Design review of the part built by this model. Coordinates are the model's own, in mm. A direction names the side the tool comes from. Give positions to 0.01 mm unless a question says otherwise; leave off trailing zeros. Loops run counter-clockwise (first coordinate to the right, second up) from the corner with the lowest first, then second, coordinate; pieces in that order, holes last. Notation, with made-up numbers: (-15, -11) -> (5, -11) arc R36 ccw to (5, 28) -> close; hole circle Ø2 at (78, 89.5). An arc over 180 degrees is marked (long way). Answer in a Markdown table with one row per item. Add a question column.
(1) For pin 1 (5.5 mm diameter, centred on y = 76, z = 12.5, fed in from -X); pin 2 (3.5 mm diameter, centred on x = 15, z = 2, fed in from +Y); pin 3 (13 mm diameter, centred on x = 26, y = 84, fed in from -Z), all flat-tipped, find the tip position at first contact; note any pin that passes through.
(2) Draft analysis for pull direction X (two halves, no side actions). For faces 4 (the flat face through (12.1, 101.5, 7)), 5 (the flat face through (0, 44, 9)), 6 (the cylindrical face through (27.2, 50.5, 8.1)), 7 (the flat face through (37, 5, 9.6)), state which applies: +X half, -X half, draft (parallel to the pull), parting line (faces both ways), or undercut.
(3) Consider section A-A on y = 41.25. Write out the cut boundary in (x, z), then the cut area to 4 significant figures.
(4) For faces 1 (the cylindrical face through (12.27, 9, 12.34)), 2 (the flat face through (21, 27, 0)), 3 (the cylindrical face through (21.492, 79.003, 10.944)), list the 3-axis set-ups (+Z, -Z, +X, -X, +Y, -Y) from which the entire face can be reached by the end or side of a thin tool; tool diameter is ignored.
(5) Consider section B-B on z = 2.5. Write out the cut boundary in (x, y).
(6) For line 1 (X direction, y = 76.5, z = 12); line 2 (Y direction, x = 21, z = 5.75); line 3 (Y direction, x = 29, z = 8.5), list the stretches that pass through material, from the lowest coordinate up.
(7) Consider section C-C on x = 21. Write out the cut boundary in (y, z).
(8) Consider section D-D on y = 7.5. Write out the cut boundary in (x, z).
from build123d import *

# Parameters (mm, degrees)
SKIZZE1_W                                            = 42.5
SKIZZE1_H                                            = 115
AUFSATZ_LINEAR_AUSTRAGEN1_DEPTH                      = 15
SKIZZE2_R                                            = 11
SCHNITT_LINEAR_AUSTRAGEN1_DEPTH                      = 14
SKIZZE3_R                                            = 9
SCHNITT_LINEAR_AUSTRAGEN2_DEPTH                      = 14
STIRNSENKUNG_F_R_M5_ZYLINDERSCHRAUBE_MIT_D           = 5.5
STIRNSENKUNG_F_R_M5_ZYLINDERSCHRAUBE_MIT_CBORE_D     = 10
STIRNSENKUNG_F_R_M5_ZYLINDERSCHRAUBE_MIT_CBORE_DEPTH = 5.4
SKIZZE6_W                                            = 7
SKIZZE6_H                                            = 47.5
SCHNITT_LINEAR_AUSTRAGEN3_DEPTH                      = 50


with BuildPart() as part:
    # Skizze1 → Aufsatz-Linear austragen1 (new body)
    with BuildSketch(Plane.XY):
        with Locations((21.25, 57.5)):
            Rectangle(SKIZZE1_W, SKIZZE1_H)
        with BuildLine():
            Line((32.25, 95), (32.25, 90))
            ThreePointArc((32.25, 90), (21.25, 79), (10.25, 90))
            Line((10.25, 90), (10.25, 95))
            ThreePointArc((10.25, 95), (21.25, 106), (32.25, 95))
        make_face(mode=Mode.SUBTRACT)
        with BuildLine():
            Line((7.5, 110.5), (7.5, 105.5))
            ThreePointArc((7.5, 105.5), (5.75, 103.75), (4, 105.5))
            Line((4, 105.5), (4, 110.5))
            ThreePointArc((4, 110.5), (5.75, 112.25), (7.5, 110.5))
        make_face(mode=Mode.SUBTRACT)
        with BuildLine():
            Line((38.5, 110.5), (38.5, 105.5))
            ThreePointArc((38.5, 105.5), (36.75, 103.75), (35, 105.5))
            Line((35, 105.5), (35, 110.5))
            ThreePointArc((35, 110.5), (36.75, 112.25), (38.5, 110.5))
        make_face(mode=Mode.SUBTRACT)
        with BuildLine():
            Line((38.5, 79.5), (38.5, 74.5))
            ThreePointArc((38.5, 74.5), (36.75, 72.75), (35, 74.5))
            Line((35, 74.5), (35, 79.5))
            ThreePointArc((35, 79.5), (36.75, 81.25), (38.5, 79.5))
        make_face(mode=Mode.SUBTRACT)
        with BuildLine():
            Line((7.5, 79.5), (7.5, 74.5))
            ThreePointArc((7.5, 74.5), (5.75, 72.75), (4, 74.5))
            Line((4, 74.5), (4, 79.5))
            ThreePointArc((4, 79.5), (5.75, 81.25), (7.5, 79.5))
        make_face(mode=Mode.SUBTRACT)
    extrude(amount=AUFSATZ_LINEAR_AUSTRAGEN1_DEPTH)

    # Skizze2 → Schnitt-Linear austragen1 (cut)
    with BuildSketch(Plane.XY.offset(15)):
        with Locations((21.25, 41.25)):
            Circle(SKIZZE2_R)
    extrude(amount=-SCHNITT_LINEAR_AUSTRAGEN1_DEPTH, mode=Mode.SUBTRACT)

    # Skizze3 → Schnitt-Linear austragen2 (cut)
    with BuildSketch(Plane.XY.offset(1)):
        with Locations((21.25, 41.25)):
            Circle(SKIZZE3_R)
    extrude(amount=-SCHNITT_LINEAR_AUSTRAGEN2_DEPTH, mode=Mode.SUBTRACT)

    # Stirnsenkung für M5 Zylinderschraube mit Innensechskant1 (through all)
    with Locations(Plane(origin=(35, 7.5, 15), x_dir=(1, 0, 0), z_dir=(0, 0, 1))):
        with Locations((0, 0), (-27.5, 0)):
            CounterBoreHole(STIRNSENKUNG_F_R_M5_ZYLINDERSCHRAUBE_MIT_D / 2, STIRNSENKUNG_F_R_M5_ZYLINDERSCHRAUBE_MIT_CBORE_D / 2, STIRNSENKUNG_F_R_M5_ZYLINDERSCHRAUBE_MIT_CBORE_DEPTH)

    # Skizze6 → Schnitt-Linear austragen3 (cut)
    with BuildSketch(Plane(origin=(42.5, 0, 0), x_dir=(0, 0, -1), z_dir=(1, 0, 0))):
        with Locations((-3.5, 91.25)):
            Rectangle(SKIZZE6_W, SKIZZE6_H)
    extrude(amount=-SCHNITT_LINEAR_AUSTRAGEN3_DEPTH, mode=Mode.SUBTRACT)


solid = part.part
Values follow:
| question | item | result |
|---|---|---|
| 1 | pin 1 | x = 0 |
| 1 | pin 2 | y = 67.5 |
| 1 | pin 3 | z = 7 |
| 2 | face 4 | draft |
| 2 | face 5 | -X half |
| 2 | face 6 | undercut |
| 2 | face 7 | undercut |
| 3 | outline | (0, 0) -> (12.25, 0) -> (12.25, 1) -> (10.25, 1) -> (10.25, 15) -> (0, 15) -> close; (30.25, 0) -> (42.5, 0) -> (42.5, 15) -> (32.25, 15) -> (32.25, 1) -> (30.25, 1) -> close |
| 3 | area | 311.5 mm2 |
| 4 | face 1 | +Z |
| 4 | face 2 | -Z, +X, -X, +Y, -Y |
| 4 | face 3 | +Z, -Z |
| 5 | outline | (0, 0) -> (42.5, 0) -> (42.5, 67.5) -> (0, 67.5) -> close; hole circle Ø5.5 at (7.5, 7.5); hole circle Ø22 at (21.25, 41.25); hole circle Ø5.5 at (35, 7.5) |
| 6 | line 1 | 0 to 4, 7.5 to 35, 38.5 to 42.5 |
| 6 | line 2 | 0 to 30.25, 52.25 to 67.5 |
| 6 | line 3 | 0 to 33.44, 49.06 to 82.19, 102.81 to 115 |
| 7 | outline | (0, 0) -> (32.25, 0) -> (32.25, 1) -> (30.25, 1) -> (30.25, 15) -> (0, 15) -> close; (50.25, 0) -> (67.5, 0) -> (67.5, 7) -> (79, 7) -> (79, 15) -> (52.25, 15) -> (52.25, 1) -> (50.25, 1) -> close; (106, 7) -> (115, 7) -> (115, 15) -> (106, 15) -> close |
| 8 | outline | (0, 0) -> (4.75, 0) -> (4.75, 9.6) -> (2.5, 9.6) -> (2.5, 15) -> (0, 15) -> close; (10.25, 0) -> (32.25, 0) -> (32.25, 9.6) -> (30, 9.6) -> (30, 15) -> (12.5, 15) -> (12.5, 9.6) -> (10.25, 9.6) -> close; (37.75, 0) -> (42.5, 0) -> (42.5, 15) -> (40, 15) -> (40, 9.6) -> (37.75, 9.6) -> close |
